Work out the finished part from the listing and answer in its coordinate system (mm). A direction names the side the tool comes from. Give positions to 0.01 mm unless a question says otherwise; leave off trailing zeros. Loops run counter-clockwise (first coordinate to the right, second up) from the corner with the lowest first, then second, coordinate; pieces in that order, holes last. Notation, with made-up numbers: (35, 21) - (67, 21) arc R13 ccw to (67, 25) - close; hole circle Ø8 at (72.5, -18). An arc over 180 degrees is marked (long way). One line per item, written item: value.
from build123d import *

# Parameters (mm, degrees)
SKETCH_1_R      = 1.000011627
SKETCH_1_R_2    = 1.000010171
SKETCH_1_R_3    = 1.000011034
SKETCH_1_R_4    = 1
EXTRUDE_1_DEPTH = 3


with BuildPart() as part:
    # 草图1 → 凸台-拉伸1 (new body)
    with BuildSketch(Plane.XY):
        with BuildLine():
            Line((28.616000433, -12.942129643), (28.616000433, -7.942129643))
            Line((28.616000433, -7.942129643), (7.141456549, -7.942129643))
            Line((7.141456549, -7.942129643), (-4.721197167, 12.792497513))
            Line((-4.721197167, 12.792497513), (-26.213755395, 12.792497513))
            ThreePointArc((-26.213755395, 12.792497513), (-28.647529033, 10.358723875), (-26.213755395, 7.924950238))
            Line((-26.213755395, 7.924950238), (-8.773244901, 7.924950238))
            Line((-8.773244901, 7.924950238), (3.165187405, -12.942129643))
            Line((3.165187405, -12.942129643), (28.616000433, -12.942129643))
        make_face()
        with Locations((5.786244634, -10.442129643)):
            Circle(SKETCH_1_R, mode=Mode.SUBTRACT)
        with Locations((14.786244634, -10.442129643)):
            Circle(SKETCH_1_R_2, mode=Mode.SUBTRACT)
        with Locations((23.786244634, -10.442129643)):
            Circle(SKETCH_1_R_3, mode=Mode.SUBTRACT)
        with Locations((-26.213755395, 10.358723875)):
            Circle(SKETCH_1_R_4, mode=Mode.SUBTRACT)
    extrude(amount=EXTRUDE_1_DEPTH)


solid = part.part
1. Flat-ended cylindrical pins translate along their axes: pin 1 Ø1.6 at (x, y) = (-26.21, 10.36) entering from -Z; pin 2 Ø1 at (y, z) = (-2.5, 0.5) entering from -X (3 decimals). Find the tip coordinate at first contact, or state that the pin passes through.
Output:
pin 1: passes through
pin 2: stops at x = -3.095
2. Find the intervals of material crossed by line 1 along Y through (x, z) = (-11, 2.8); line 2 along Y through (x, z) = (12, 0.6); line 3 along Y through (x, z) = (6.5, 2.55), in increasing order.
Output:
line 1: y = 7.92 to 12.79
line 2: y = -12.94 to -7.94
line 3: y = -12.94 to -11.14, -9.74 to -6.82
3. Section B-B (z = 0.8) is taken. Write down the section's boundary in (x, y), and give its area (3 significant figures).
Output:
outline: (-26.21, 7.92) - (-8.77, 7.92) - (3.17, -12.94) - (28.62, -12.94) - (28.62, -7.94) - (7.14, -7.94) - (-4.72, 12.79) - (-26.21, 12.79) arc R2.43 ccw to start; hole circle Ø2 at (-26.21, 10.36); hole circle Ø2 at (5.79, -10.44); hole circle Ø2 at (14.79, -10.44); hole circle Ø2 at (23.79, -10.44)
area: 351 mm²
4. The mould has two halves that part along X. Classify faces 4 (the flat face through (28.616, -10, 1)), 5 (the cylindrical face through (13.787, -10.398, 1.479)), 6 (the flat face through (-15, 12.792, 1)): released by +X, released by -X, zero draft, split by the parting line, or undercut.
Output:
face 4: released by +X
face 5: undercut
face 6: zero draft
5. Section A-A (x = 17) is taken. Write down the section's boundary in (y, z).
Output:
outline: (-12.94, 0) - (-7.94, 0) - (-7.94, 3) - (-12.94, 3) - close
6. For faces 1 (the cylindrical face through (-28.647, 10.412, 1.479)), 2 (the flat face through (-18, 7.925, 1)), 3 (the flat face through (18, -7.942, 1)), determine the directions among +Z, -Z, +X, -X, +Y, -Y from which every point of the face is accessible in a straight line to the end or side of a thin tool.
Output:
face 1: +Z, -Z, -X
face 2: +Z, -Z, -X, -Y
face 3: +Z, -Z, +X, +Y
7. Section C-C (y = 3) is taken. Write down the section's boundary in (x, z).
Output:
outline: (-5.96, 0) - (0.88, 0) - (0.88, 3) - (-5.96, 3) - close
